The listing builds one solid part. Answer for the finished solid, in the listing's coordinates (mm). Face numbers are marked on the shaded views. Coordinates: 2 decimals unless noted, no trailing zeros. Order: outer loops, then holes, each group sorted by start corner. A loop starts at its lowest first (then second) coordinate and runs counter-clockwise, first axis right, second up.
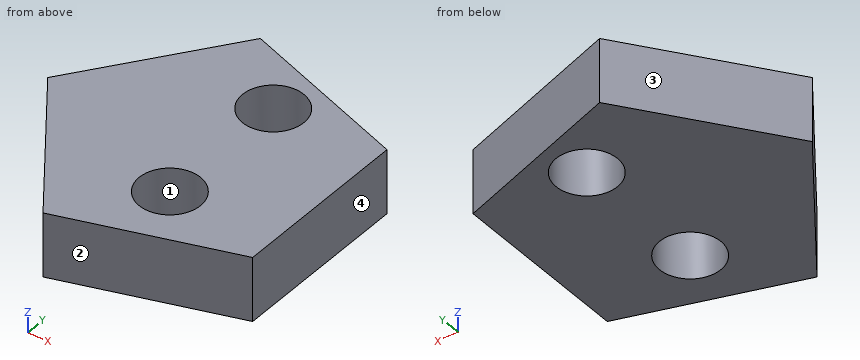
from build123d import *

# Parameters (mm, degrees)
F1_DEPTH = 25.4
F3_D     = 24.20874


with BuildPart() as f1:
    # F0 (on Top) → F1 (new body)
    with BuildSketch(Plane.XY):
        Polygon((48.0459555984, -34.9074300409), (48.0459555984, 34.9074300409), (-18.3519220166, 56.481408266), (-59.3880671635, 0), (-18.3519220166, -56.481408266), align=None)
    extrude(amount=F1_DEPTH)

    # F3 (through all)
    with Locations(Plane(origin=(0, 0, 0), x_dir=(1, 0, 0), z_dir=(0, 0, -1))):
        with Locations((6.7180017941, 23.5614608973), (6.7180017941, -30.1724821329)):
            Hole(F3_D / 2)


solid = f1.part
1) Each of these flat-tipped pins is pushed along its axis until it touches: P1, Ø12, axis at x = -41, z = 12, coming from the -Y side; P2, Ø14.5, axis at x = 6.72, y = 30.17, coming from the +Z side (3 decimals); P3, Ø1.5, axis at x = -0.5, z = 15, coming from the +Y side; P4, Ø10, axis at x = 9.5, z = 2.5, coming from the +Y side. Where does it stop, or does it pass through?
2) Determine the mould class of the marked faces 1, 2, 3 and 4 for opening direction Y: released by +Y, released by -Y, zero draft, split by the parting line, or undercut.
3) Section A-A (x = 9.5) is taken. Give the vertices of the cut face in (y, z).
4) Section B-B (y = -33.5) is taken. Give the vertices of the cut face in (x, z).
5) Section C-C (z = 13.5) is taken. Give the vertices of the cut face in (x, y), then the cut area to 3 significant figures.
6) Consider L1, parallel to Y at x = 5, z = 21.75; L2, parallel to Y at x = 2, z = 1; L3, parallel to X at y = 28, z = 15. Determine where each line is inside the solid, lowest interval first.
7) Section D-D (x = -40) is taken. Give the vertices of the cut face in (y, z), then the cut area to 3 significant figures.
Filled sheet:
1. P1: stops at y = -33.57
1. P2: passes through
1. P3: stops at y = 50.92
1. P4: stops at y = 49.06
2. face 1: undercut
2. face 2: released by -Y
2. face 3: released by +Y
2. face 4: zero draft
3. outline: (-47.43, 0) - (-35.34, 0) - (-35.34, 25.4) - (-47.43, 25.4) - close; (-11.78, 0) - (18.39, 0) - (18.39, 25.4) - (-11.78, 25.4) - close; (41.95, 0) - (47.43, 0) - (47.43, 25.4) - (41.95, 25.4) - close
4. outline: (-35.05, 0) - (-0.19, 0) - (-0.19, 25.4) - (-35.05, 25.4) - close; (13.63, 0) - (48.05, 0) - (48.05, 25.4) - (13.63, 25.4) - close
5. outline: (-59.39, 0) - (-18.35, -56.48) - (48.05, -34.91) - (48.05, 34.91) - (-18.35, 56.48) - close; hole circle Ø24.21 at (6.72, -23.56); hole circle Ø24.21 at (6.72, 30.17)
5. area: 7,470 mm2
6. L1: y = -48.89 to -35.54, -11.58 to 18.19, 42.15 to 48.89
6. L2: y = -49.87 to -34.71, -12.41 to 19.03, 41.32 to 49.87
6. L3: x = -39.04 to -5.19, 18.63 to 48.05
7. outline: (-26.69, 0) - (26.69, 0) - (26.69, 25.4) - (-26.69, 25.4) - close
7. area: 1,360 mm2
